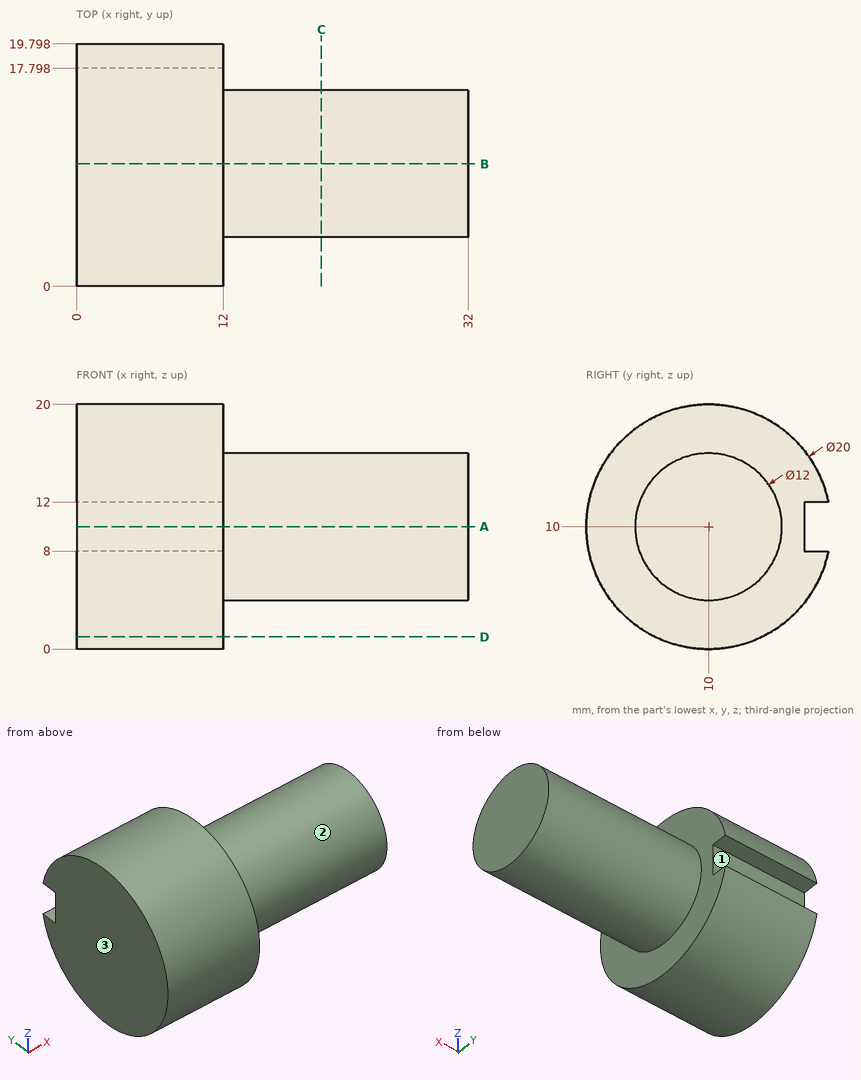
For this review, use the dimensioned drawing (mm, ordinates from the lowest corner) and the shaded views. A direction names the side the tool comes from. Round coordinates to 2 decimals unless told otherwise and drop trailing zeros. Write each loop counter-clockwise with the first axis right and the second up, starting at its lowest first coordinate (ties: lowest second). Pieces come first, ordered by that corner, then holes. Notation, with made-up numbers: M -18,-17.5 L 29,-17.5 A17 ccw 29,10.5 Z; hole C -11,30 d4. An arc over 180 degrees is marked long. Use CSV: the item, a comma, the result in double quotes. Start each with the question number.
(1) We need section C-C, the plane x = 20. State the section outline as (y, z) points, then the cut area to 3 significant figures.
(2) Clearance check with flat-ended pins moving along their axes: P1, Ø6, axis at x = 6.5, y = 5.5, coming from the -Z side; P2, Ø3, axis at x = 15.5, y = 16, coming from the +Z side; P3, Ø1, axis at x = 5.5, y = 19, coming from the +Z side. State where each tip first meets the part, or that it passes through.
(3) We need section A-A, the plane z = 10. State the section outline as (x, y) points.
(4) For line 1 along Z through (x, y) = (10, 9.75); line 2 along X through (y, z) = (5, 4); line 3 along Y through (x, z) = (7, 4.5), list the stretches that pass through material, from the lowest coordinate up.
(5) We need section D-D, the plane z = 1. State the section outline as (x, y) points, then the cut area to 3 significant figures.
(6) We need section B-B, the plane y = 10. State the section outline as (x, z) points, then the cut area to 3 significant figures.
(7) Tool access review of the marked faces 1, 2 and 3: name each direction out of +Z, -Z, +X, -X, +Y, -Y from which nothing blocks a thin tool from reaching the whole face with its end or side.
Findings:
1,outline,"C 10,10 d12"
1,area,"113 mm^2"
2,P1,"z = 0.11"
2,P2,"z = 13.97"
2,P3,"z = 15.27"
3,outline,"M 0,0 L 12,0 L 12,4 L 32,4 L 32,16 L 12,16 L 12,17.8 L 0,17.8 Z"
4,line 1,"0 to 20"
4,line 2,"0 to 12"
4,line 3,"1.65 to 18.35"
5,outline,"M 0,5.64 L 12,5.64 L 12,14.36 L 0,14.36 Z"
5,area,"105 mm^2"
6,outline,"M 0,0 L 12,0 L 12,4 L 32,4 L 32,16 L 12,16 L 12,20 L 0,20 Z"
6,area,"480 mm^2"
7,face 1,"+X, -X, +Y"
7,face 2,"+X"
7,face 3,"+Z, -Z, -X, +Y, -Y"
